Source: CAD feature listing. Evaluate the final solid. Frame: model axes, mm. A direction names the side the tool comes from. Round coordinates to 2 decimals unless told otherwise and drop trailing zeros. Write each loop counter-clockwise with the first axis right and the second up, starting at its lowest first coordinate (ties: lowest second). Pieces come first, ordered by that corner, then holes.
from build123d import *

# Parameters (mm, degrees)
PAD009_DEPTH    = 8
POCKET005_DEPTH = 6
SKETCH044_W     = 20
SKETCH044_H     = 15
PAD010_DEPTH    = 3
SKETCH045_R     = 1.45
POCKET006_DEPTH = 149.538323
SKETCH046_W     = 10
SKETCH046_H     = 20
POCKET007_DEPTH = 6
SKETCH047_W     = 5
SKETCH047_H     = 8
PAD011_DEPTH    = 4
PAD012_DEPTH    = 3


with BuildPart() as part:
    # Sketch042 → Pad009 (new body)
    with BuildSketch(Plane.XY):
        with BuildLine():
            ThreePointArc((14.331049, 53.958076), (14.329401, 54.015983), (14.328712, 54.073909))
            Line((14.131233, 108.554683), (14.328712, 54.073909))
            ThreePointArc((14.131233, 108.554683), (14.131214, 108.572623), (14.131287, 108.590561))
            ThreePointArc((18.658021, 113.117293), (15.46591, 111.782672), (14.131287, 108.590561))
            ThreePointArc((18.658021, 113.117293), (18.669616, 113.117351), (18.681211, 113.11737))
            Line((101.94388, 113.11737), (18.681211, 113.11737))
            ThreePointArc((101.94388, 113.11737), (101.963094, 113.117317), (101.982307, 113.117159))
            Line((113.720987, 112.988269), (101.982307, 113.117159))
            ThreePointArc((113.720987, 112.988269), (113.760941, 112.987602), (113.800884, 112.986479))
            Line((124.730854, 112.616759), (113.800884, 112.986479))
            ThreePointArc((124.730854, 112.616759), (124.775077, 112.614983), (124.819274, 112.612649))
            Line((134.707394, 112.027539), (124.819274, 112.612649))
            ThreePointArc((134.707394, 112.027539), (134.760897, 112.023961), (134.814338, 112.019564))
            Line((143.427438, 111.244494), (134.814338, 112.019564))
            ThreePointArc((143.427438, 111.244494), (143.500111, 111.23719), (143.572616, 111.22837))
            Line((150.677556, 110.28877), (143.572616, 111.22837))
            ThreePointArc((150.677556, 110.28877), (150.793483, 110.271459), (150.908765, 110.250277))
            Line((156.272395, 109.171587), (150.908765, 110.250277))
            ThreePointArc((156.272395, 109.171587), (156.5104, 109.115), (156.743872, 109.041926))
            Line((160.133022, 107.849586), (156.743872, 109.041926))
            ThreePointArc((160.133022, 107.849586), (160.895244, 107.471834), (161.543817, 106.92135))
            Line((162.725347, 105.64078), (161.543817, 106.92135))
            ThreePointArc((162.725347, 105.64078), (163.413102, 104.540852), (163.653, 103.265981))
            Line((163.653, 103.265981), (163.62255, 27.110501))
            ThreePointArc((163.62255, 27.110501), (163.60451, 26.756997), (163.550857, 26.407123))
            ThreePointArc((159.660239, 22.516538), (162.188858, 23.878516), (163.550857, 26.407123))
            ThreePointArc((159.660239, 22.516538), (159.323063, 22.464205), (158.982393, 22.444954))
            Line((158.982393, 22.444954), (158.507799, 22.441306))
            ThreePointArc((158.507799, 22.441306), (158.494348, 22.441228), (158.480896, 22.441202))
            Line((116.551548, 22.441202), (158.480896, 22.441202))
            ThreePointArc((116.551548, 22.441202), (116.524186, 22.427455), (116.51234, 22.399217))
            Line((116.51234, 22.399217), (116.51234, 12.693214))
            ThreePointArc((111.511608, 7.69248), (115.048134, 9.156687), (116.51234, 12.693214))
            Line((53.496079, 7.69248), (111.511608, 7.69248))
            Line((40.903121, 0.40324), (53.496079, 7.69248))
            ThreePointArc((40.903121, 0.40324), (40.82134, 0.357354), (40.738359, 0.313675))
            Line((40.570469, 0.228155), (40.738359, 0.313675))
            ThreePointArc((40.570469, 0.228155), (40.28044, 0.096677), (39.97966, -0.007897))
            Line((39.821, -0.055087), (39.97966, -0.007897))
            ThreePointArc((39.821, -0.055087), (39.4375, -0.145999), (39.04621, -0.193218))
            Line((38.89726, -0.202728), (39.04621, -0.193218))
            ThreePointArc((38.89726, -0.202728), (38.443297, -0.202212), (37.99322, -0.142943))
            Line((37.85444, -0.115413), (37.99322, -0.142943))
            ThreePointArc((37.85444, -0.115413), (37.403892, 0.005662), (36.973449, 0.185583))
            Line((36.845299, 0.249493), (36.973449, 0.185583))
            ThreePointArc((36.845299, 0.249493), (36.477576, 0.461653), (36.138245, 0.716774))
            Line((36.021215, 0.816424), (36.138245, 0.716774))
            ThreePointArc((36.021215, 0.816424), (35.764889, 1.057957), (35.534135, 1.324028))
            Line((35.428675, 1.458768), (35.534135, 1.324028))
            ThreePointArc((35.428675, 1.458768), (35.268511, 1.680768), (35.126187, 1.914607))
            Line((35.047407, 2.056233), (35.126187, 1.914607))
            Line((21.664757, 24.948224), (35.047407, 2.056233))
            ThreePointArc((21.664757, 24.948224), (21.600836, 25.062414), (21.541228, 25.178913))
            ThreePointArc((14.331049, 53.958076), (16.428723, 39.190834), (21.541228, 25.178913))
        make_face()
    extrude(amount=PAD009_DEPTH)

    # Sketch043 → Pocket005 (cut)
    with BuildSketch(Plane.XY):
        with BuildLine():
            ThreePointArc((17.329026, 54.068236), (19.338784, 39.919906), (24.237019, 26.495239))
            ThreePointArc((24.254666, 26.462283), (24.245534, 26.478596), (24.237019, 26.495239))
            Line((24.254666, 26.462283), (37.653506, 3.542597))
            Line((37.653506, 3.542597), (37.747881, 3.372935))
            ThreePointArc((37.791094, 3.307815), (37.768213, 3.33953), (37.747881, 3.372935))
            Line((37.791094, 3.307815), (37.896554, 3.173075))
            ThreePointArc((37.966136, 3.100561), (37.929518, 3.135065), (37.896554, 3.173075))
            Line((37.966136, 3.100561), (38.083166, 3.000911))
            ThreePointArc((38.184174, 2.934156), (38.131642, 2.964465), (38.083166, 3.000911))
            Line((38.184174, 2.934156), (38.312324, 2.870246))
            ThreePointArc((38.43818, 2.827247), (38.373816, 2.844543), (38.312324, 2.870246))
            Line((38.43818, 2.827247), (38.57696, 2.799717))
            ThreePointArc((38.706109, 2.791176), (38.641257, 2.79125), (38.57696, 2.799717))
            Line((38.706109, 2.791176), (38.855059, 2.800686))
            ThreePointArc((38.965743, 2.820419), (38.910957, 2.807432), (38.855059, 2.800686))
            Line((38.965743, 2.820419), (39.124403, 2.867609))
            ThreePointArc((39.208804, 2.901331), (39.167371, 2.882548), (39.124403, 2.867609))
            Line((39.208804, 2.901331), (39.376694, 2.986851))
            ThreePointArc((39.400232, 2.999646), (39.388549, 2.993091), (39.376694, 2.986851))
            Line((39.400232, 2.999646), (52.690443, 10.69248))
            Line((52.690443, 10.69248), (111.512203, 10.69248))
            ThreePointArc((111.512203, 10.69248), (112.926813, 11.278007), (113.51234, 12.692618))
            Line((113.51234, 22.413147), (113.51234, 12.692618))
            ThreePointArc((116.515571, 25.441202), (114.395073, 24.540983), (113.51234, 22.413147))
            Line((116.515571, 25.441202), (158.480896, 25.441202))
            ThreePointArc((158.484739, 25.441217), (158.482818, 25.441206), (158.480896, 25.441202))
            Line((158.959333, 25.444865), (158.484739, 25.441217))
            ThreePointArc((159.056169, 25.455091), (159.008, 25.447615), (158.959333, 25.444865))
            ThreePointArc((159.056169, 25.455091), (160.067546, 25.999845), (160.612308, 27.011218))
            ThreePointArc((160.62255, 27.111701), (160.619973, 27.0612), (160.612308, 27.011218))
            Line((160.653, 103.26718), (160.62255, 27.111701))
            ThreePointArc((160.520478, 103.606437), (160.618729, 103.449305), (160.653, 103.26718))
            Line((160.520478, 103.606437), (159.338948, 104.887007))
            ThreePointArc((159.137406, 105.019612), (159.246295, 104.965648), (159.338948, 104.887007))
            Line((159.137406, 105.019612), (155.748256, 106.211952))
            ThreePointArc((155.680902, 106.230475), (155.714903, 106.222391), (155.748256, 106.211952))
            Line((155.680902, 106.230475), (150.317272, 107.309165))
            ThreePointArc((150.284242, 107.314664), (150.300803, 107.312191), (150.317272, 107.309165))
            Line((150.284242, 107.314664), (143.179302, 108.254264))
            ThreePointArc((143.158563, 108.256568), (143.168944, 108.255524), (143.179302, 108.254264))
            Line((143.158563, 108.256568), (134.545463, 109.031638))
            ThreePointArc((134.530185, 109.032777), (134.537828, 109.032266), (134.545463, 109.031638))
            Line((134.530185, 109.032777), (124.642065, 109.617887))
            ThreePointArc((124.629433, 109.618474), (124.635751, 109.61822), (124.642065, 109.617887))
            Line((124.629433, 109.618474), (113.699463, 109.988194))
            ThreePointArc((113.68805, 109.98845), (113.693757, 109.988355), (113.699463, 109.988194))
            Line((113.68805, 109.98845), (101.94937, 110.11734))
            ThreePointArc((101.94388, 110.11737), (101.946625, 110.117362), (101.94937, 110.11734))
            Line((101.94388, 110.11737), (18.681211, 110.11737))
            ThreePointArc((18.677898, 110.117359), (18.679554, 110.117367), (18.681211, 110.11737))
            ThreePointArc((18.677898, 110.117359), (17.58723, 109.661351), (17.131221, 108.570683))
            ThreePointArc((17.131213, 108.565558), (17.131211, 108.56812), (17.131221, 108.570683))
            Line((17.131213, 108.565558), (17.328692, 54.084784))
            ThreePointArc((17.329026, 54.068236), (17.328791, 54.076508), (17.328692, 54.084784))
        make_face()
    extrude(amount=POCKET005_DEPTH, mode=Mode.SUBTRACT)

    # Sketch044 → Pad010 (new body)
    with BuildSketch(Plane(origin=(14.524525, 0.052648, 0), x_dir=(0.003625, -0.999993, 0), z_dir=(-0.999993, -0.003625, 0))):
        with Locations((-75.54892, 0.5)):
            Rectangle(SKETCH044_W, SKETCH044_H)
    extrude(amount=-PAD010_DEPTH)

    # Sketch045 (on Face112 of Pad010) → Pocket006 (cut, through all)
    with BuildSketch(Plane(origin=(14.524525, 0.052648, 0), x_dir=(0.003625, -0.999993, 0), z_dir=(-0.999993, -0.003625, 0))):
        with Locations((-75.54892, -2.25)):
            Circle(SKETCH045_R)
    extrude(amount=-POCKET006_DEPTH, mode=Mode.SUBTRACT)

    # Sketch046 (on Face3 of Pocket006) → Pocket007 (cut)
    with BuildSketch(Plane(origin=(14.524525, 0.052648, 0), x_dir=(0.003625, -0.999993, 0), z_dir=(-0.999993, -0.003625, 0))):
        with Locations((-43.04892, -2)):
            Rectangle(SKETCH046_W, SKETCH046_H)
    extrude(amount=-POCKET007_DEPTH, mode=Mode.SUBTRACT)

    # Sketch047 (on Face3 of Pocket007) → Pad011 (new body)
    with BuildSketch(Plane(origin=(14.524525, 0.052648, 0), x_dir=(0.003625, -0.999993, 0), z_dir=(-0.999993, -0.003625, 0))):
        with Locations((-35.54892, 4)):
            Rectangle(SKETCH047_W, SKETCH047_H)
    extrude(amount=-PAD011_DEPTH)

    # Sketch047 (on Face3 of Pocket007) → Pad012 (new body)
    with BuildSketch(Plane(origin=(14.524525, 0.052648, 0), x_dir=(0.003625, -0.999993, 0), z_dir=(-0.999993, -0.003625, 0))):
        with Locations((-35.54892, 4)):
            Rectangle(SKETCH047_W, SKETCH047_H)
    extrude(amount=PAD012_DEPTH)


solid = part.part
1) Material intervals for line 1 (X direction, y = 88.5, z = 5); line 2 (Z direction, x = 80.5, y = 26.5); line 3 (X direction, y = 84, z = -1), sorted ascending.
Taken from the geometry:
line 1: x = 14.2 to 17.2, 160.65 to 163.65
line 2: z = 6 to 8
line 3: x = 14.22 to 17.22
2) Pull-direction query (Y, two-part tool) for faces 1 (the face through (137, 22.441, 4)), 2 (the face through (114.418, 24.564, 2.958)), 3 (the face through (158.46, 108.44, 3.94)); classes: released by +Y, released by -Y, zero draft, split by the parting line, or undercut.
Taken from the geometry:
face 1: released by -Y
face 2: undercut
face 3: released by +Y
3) Section query C-C on z = -5.25. Return the cut outline in (x, y).
Taken from the geometry:
outline: (14.21, 85.6) - (14.29, 65.6) - (17.29, 65.61) - (17.21, 85.61) - close
4) Reachability of faces 4 (the face through (116.512, 18, 4)), 5 (the face through (139.181, 111.627, 3.944)), 6 (the face through (129.66, 109.32, 2.96)) from +Z, -Z, +X, -X, +Y, -Y: full face, straight path, thin tool, end or side. Return the list, or none.
Taken from the geometry:
face 4: +Z, -Z, +X, -Y
face 5: +Z, -Z, +X, +Y
face 6: -Z
5) Contact query for flat-ended pins moving along their axis: P1, Ø5, axis at x = 64.5, z = -1.5, coming from the -Y side; P2, Ø10, axis at x = 124, y = 44.5, coming from the -Z side; P3, Ø5, axis at x = 127.5, z = 4.5, coming from the +Y side. Output: stop coordinate, or through.
Taken from the geometry:
P1: stops at y = 7.69
P2: stops at z = 6
P3: stops at y = 112.6
6) Section query B-B on x = 85.5. Return the cut outline in (y, z).
Taken from the geometry:
outline: (7.69, 0) - (10.69, 0) - (10.69, 6) - (110.12, 6) - (110.12, 0) - (113.12, 0) - (113.12, 8) - (7.69, 8) - close
